Source: CAD feature listing. Evaluate the final solid. Frame: model axes, mm. A direction names the side the tool comes from. Round coordinates to 2 decimals unless told otherwise and drop trailing zeros. Loops run counter-clockwise (first coordinate to the right, second up) from the corner with the lowest first, then second, coordinate; pieces in that order, holes last. Notation, with made-up numbers: M 31.5,29 L 42.5,29 A16 ccw 42.5,38 Z; hole C -24.75,69 d7. An arc over 180 degrees is marked long. Answer as CSV lines item,"result". Start each with the question number.
```python
from build123d import *

# Parameters (mm, degrees)
F1_DEPTH = 50.8
F3_DEPTH = 50.8
F4_R     = 3.175
F5_DEPTH = 50.8


with BuildPart() as f1:
    # F0 (on Front) → F1 (new body)
    with BuildSketch(Plane.XZ):
        Polygon((104.640433, 0), (80.510433, 32.204173), (56.380433, 0), (61.460433, 0), (80.510433, 25.424347), (99.560433, 0), align=None)
        Polygon((-14.149985, 35.374962), (0, 0), (80.510433, 32.204173), (161.020865, 64.408346), (156.304203, 76.2), (0, 13.678319), (-9.433323, 37.261627), align=None)
    extrude(amount=F1_DEPTH)

    # F2 (on face) → F3 (cut)
    with BuildSketch(Plane.XZ.offset(50.8)):
        Polygon((117.38383, 0), (80.510433, 32.204173), (41.978721, -5.036601), align=None)
    extrude(amount=-F3_DEPTH, mode=Mode.SUBTRACT)

    # F4 (on face) → F5 (cut)
    with BuildSketch(Plane.XZ.offset(50.8)):
        with Locations((78.152102, 38.1)):
            Circle(F4_R)
    extrude(amount=-F5_DEPTH, mode=Mode.SUBTRACT)


solid = f1.part
```
1) Contact query for flat-ended pins moving along their axis: pin 1 Ø10 at (x, y) = (123, -26) entering from +Z; pin 2 Ø1 at (x, y) = (98, -25) entering from -Z; pin 3 Ø6 at (x, y) = (120, -38.5) entering from +Z; pin 4 Ø5 at (x, z) = (78.15, 38.1) entering from +Y. Output: stop coordinate, or through.
2) Section D-D, the plane z = 54.5. Return loops of the section in (x, y), and give its area (3 significant figures).
3) Access query for faces 1 (the flat face through (-7.174, -25.044, 17.935)), 2 (the flat face through (-4.65, -25.04, 25.3)). Directions: +Z, -Z, +X, -X, +Y, -Y. A direction counts if a zero-diameter tool reaches every point of the face in a straight line with its end or side. Return the directions, or none.
4) Ray query, line 1 along Z through (x, y) = (137, -41.5); line 2 along Z through (x, y) = (10, -22.5). Return the intervals inside material, ascending.
5) Section B-B, the plane z = 30. Return loops of the section in (x, y), and give its area (3 significant figures).
6) Section A-A, the plane y = -42. Return loops of the section in (x, z) (3 decimals).
7) Mould query, pull axis X, two halves, no side actions, for faces 3 (the flat face through (79.25, -25.04, 45.38)), 4 (the flat face through (-11.76, -25.04, 36.33)), 5 (the flat face through (158.696, -25.044, 70.222)). Classes: pulls with the +X half, pulls with the -X half, needs draft (parallel to the pull), parting line crosses it, or undercut.
8) Section C-C, the plane x = 107.5. Return loops of the section in (y, z), and give its area (3 significant figures).
Findings below:
1,pin 1,"z = 64.88"
1,pin 2,"z = 39"
1,pin 3,"z = 62.88"
1,pin 4,"through"
2,outline,"M 102.05,-50.8 L 136.25,-50.8 L 136.25,0 L 102.05,0 Z"
2,area,"1,740 mm²"
3,face 1,"-Z, -X, +Y, -Y"
3,face 2,"+Z, +Y, -Y"
4,line 1,"54.8 to 68.48"
4,line 2,"4 to 17.68"
5,outline,"M -12,-50.8 L -6.53,-50.8 L -6.53,0 L -12,0 Z; M 40.8,-50.8 L 75,-50.8 L 75,0 L 40.8,0 Z"
5,area,"2,020 mm²"
6,outline,"M -14.15,35.375 L 0,0 L 161.021,64.408 L 156.304,76.2 L 0,13.678 L -9.433,37.262 Z; hole C 78.152,38.1 d6.35"
7,face 3,"undercut"
7,face 4,"pulls with the -X half"
7,face 5,"pulls with the +X half"
8,outline,"M -50.8,43 L 0,43 L 0,56.68 L -50.8,56.68 Z"
8,area,"695 mm²"
